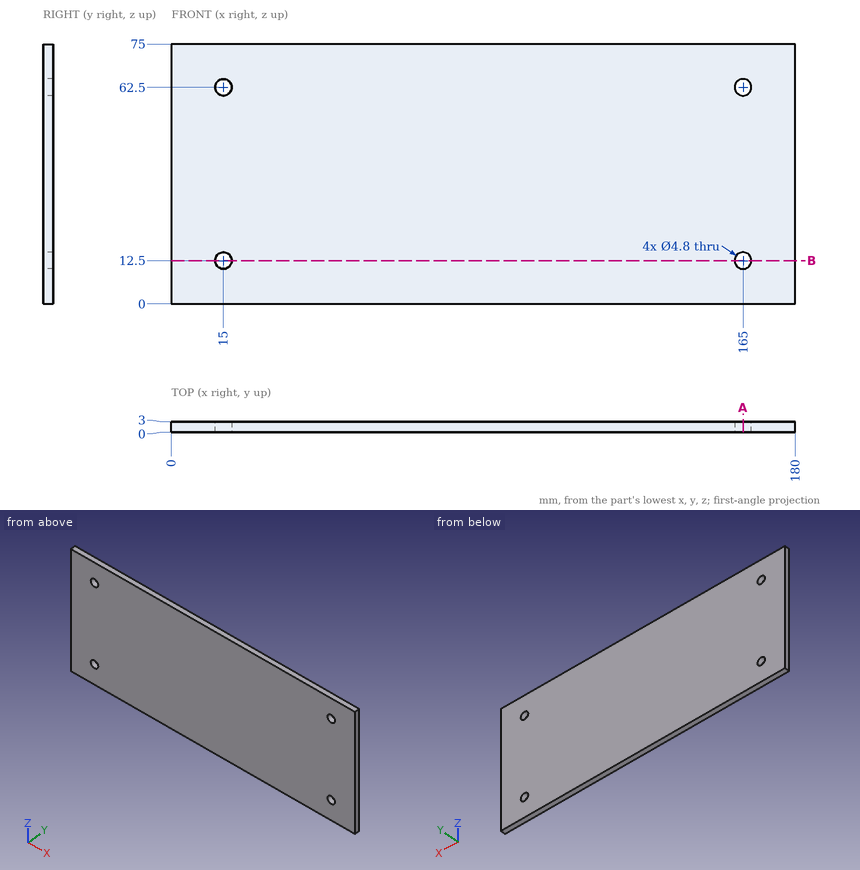
For this review, use the dimensioned drawing (mm, ordinates from the lowest corner) and the shaded views. Give positions to 0.01 mm unless a question says otherwise; leave off trailing zeros. Order: outer loops, then holes, each group sorted by start corner. A loop starts at its lowest first (then second) coordinate and runs counter-clockwise, first axis right, second up. Notation, with made-up numbers: M 24,76 L 49,76 A19 ccw 49,90 Z; hole C 21,-27 d5. An arc over 180 degrees is marked long. One line per question, with ' | ' between items. Start each with the question number.
1) Clearance check with a flat-ended pin moving along its axis: P1, Ø6, axis at x = 15, z = 62.5, coming from the -Y side. State where the tip first meets the part, or that it passes through.
2) Wall thickness on L1, parallel to Z at x = 165, y = 2.1; L2, parallel to X at y = 1.2, z = 12; L3, parallel to Z at x = 13, y = 2.8: over which ranges is each line inside the solid? List them lowest first. Write a range as from..to.
3) Consider section A-A, the plane x = 165. Give the boundary of the cut face in (y, z).
4) Consider section B-B, the plane z = 12.5. Give the boundary of the cut face in (x, y).
Found:
1) P1: stops at y = 0
2) L1: z = 0..10.1, 14.9..60.1, 64.9..75 | L2: x = 0..12.65, 17.35..162.65, 167.35..180 | L3: z = 0..11.17, 13.83..61.17, 63.83..75
3) outline: M 0,0 L 3,0 L 3,10.1 L 0,10.1 Z; M 0,14.9 L 3,14.9 L 3,60.1 L 0,60.1 Z; M 0,64.9 L 3,64.9 L 3,75 L 0,75 Z
4) outline: M 0,0 L 12.6,0 L 12.6,3 L 0,3 Z; M 17.4,0 L 162.6,0 L 162.6,3 L 17.4,3 Z; M 167.4,0 L 180,0 L 180,3 L 167.4,3 Z
